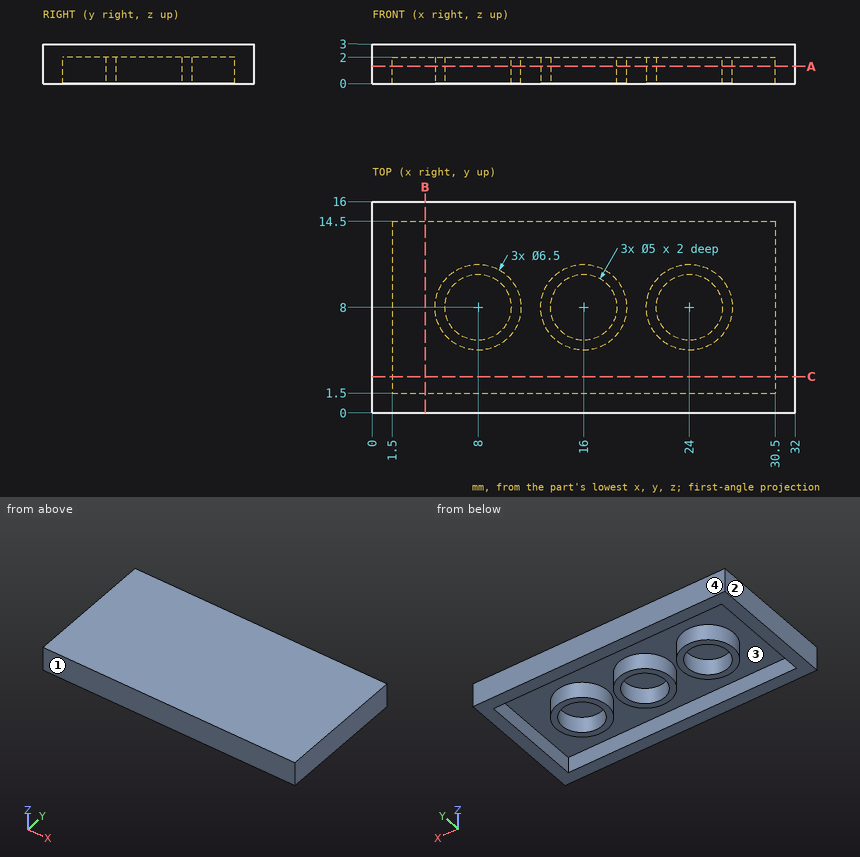
Geometry check sheet. Reference: drawing and pictorial views, mm from the part's lowest x, y, z. Round coordinates to 2 decimals unless told otherwise and drop trailing zeros. Loops run counter-clockwise (first coordinate to the right, second up) from the corner with the lowest first, then second, coordinate; pieces in that order, holes last. Notation, with made-up numbers: (13.5, 17.5) - (71.5, 17.5) arc R16 ccw to (71.5, 25.5) - close; hole circle Ø1 at (12.25, 84). An arc over 180 degrees is marked (long way). Answer as CSV lines item,"result".
(1) Cross-section at B-B, the plane x = 4. Enter the section's corners in (y, z).
Output values:
outline,"(0, 0) - (1.5, 0) - (1.5, 2) - (14.5, 2) - (14.5, 0) - (16, 0) - (16, 3) - (0, 3) - close"
(2) Release check for a two-part mould opening along Y. For the marked faces 1, 2, 3 and 4 record: released by +Y, released by -Y, zero draft, split by the parting line, or undercut.
Output values:
face 1,"released by -Y"
face 2,"zero draft"
face 3,"undercut"
face 4,"released by +Y"
(3) Cross-section at C-C, the plane y = 2.75. Enter the section's corners in (x, z).
Output values:
outline,"(0, 0) - (1.5, 0) - (1.5, 2) - (30.5, 2) - (30.5, 0) - (32, 0) - (32, 3) - (0, 3) - close"
(4) Cross-section at A-A, the plane z = 1.3. Enter the section's corners in (x, y).
Output values:
outline,"(0, 0) - (32, 0) - (32, 16) - (0, 16) - close; circle Ø6.5 at (8, 8); circle Ø6.5 at (16, 8); circle Ø6.5 at (24, 8); hole (1.5, 1.5) - (30.5, 1.5) - (30.5, 14.5) - (1.5, 14.5) - close; hole circle Ø5 at (8, 8); hole circle Ø5 at (16, 8); hole circle Ø5 at (24, 8)"
(5) Material ranges on line 1 along Y through (x, z) = (8, 1.35); line 2 along X through (y, z) = (2.75, 0.35); line 3 along Y through (x, z) = (3, 0.45), recorded low to high.
Output values:
line 1,"y = 0 to 1.5, 4.75 to 5.5, 10.5 to 11.25, 14.5 to 16"
line 2,"x = 0 to 1.5, 30.5 to 32"
line 3,"y = 0 to 1.5, 14.5 to 16"
(6) Depth check by flat-ended pin: pin 1 Ø1.5 at (x, y) = (25, 7) entering from -Z. Enter the tip coordinate at first touch or a pass-through.
Output values:
pin 1,"stops at z = 2"
